```python
from build123d import *

# Parameters (mm, degrees)
EXTRUDE_1_DEPTH     = 35
FILLET_START        = -36
FILLET_1_DEPTH      = 37
FILLET_START_2      = -35
FILLET_1_2_DEPTH    = 35
SKETCH_2_R          = 2
CUT_EXTRUDE_1_DEPTH = 40.515819617
CUT_EXTRUDE_2_DEPTH = 2.5
EXTRUDE_2_DEPTH     = 5.1


with BuildPart() as part:
    # 草图1 → 凸台-拉伸1 (new body)
    with BuildSketch(Plane.XY):
        with BuildLine():
            Line((-2, 11.5), (-2, -11.5))
            Line((-2, -11.5), (0, -11.5))
            Line((0, -11.5), (0, -14.5))
            Line((0, -14.5), (0, -17.5))
            Line((0, -17.5), (-1, -17.5))
            Line((-1, -17.5), (-1, -14.5))
            ThreePointArc((-1, -14.5), (-1.292893219, -13.792893219), (-2, -13.5))
            Line((-2, -13.5), (-3.5, -13.5))
            ThreePointArc((-3.5, -13.5), (-4.914213562, -12.914213562), (-5.5, -11.5))
            Line((-5.5, -11.5), (-5.5, 11.5))
            ThreePointArc((-5.5, 11.5), (-4.914213562, 12.914213562), (-3.5, 13.5))
            Line((-3.5, 13.5), (-2, 13.5))
            ThreePointArc((-2, 13.5), (-1.292893219, 13.792893219), (-1, 14.5))
            Line((-1, 14.5), (-1, 17.5))
            Line((-1, 17.5), (0, 17.5))
            Line((0, 17.5), (0, 14.5))
            Line((0, 14.5), (0, 11.5))
            Line((0, 11.5), (-2, 11.5))
        make_face()
    extrude(amount=-EXTRUDE_1_DEPTH)

    # 圆角1: read off the stored shape, not the designer's step
    # 圆角1 outline → 圆角1 (cut)
    with BuildSketch(Plane.XY.offset(FILLET_START)):
        with BuildLine():
            Line((0, -11.5), (-1, -11.5))
            ThreePointArc((-1, -11.5), (-0.292893219, -11.792893219), (0, -12.5))
            Line((0, -12.5), (0, -11.5))
        make_face()
        with BuildLine():
            ThreePointArc((0, 12.5), (-0.292893219, 11.792893219), (-1, 11.5))
            Line((-1, 11.5), (0, 11.5))
            Line((0, 11.5), (0, 12.5))
        make_face()
    extrude(amount=FILLET_1_DEPTH, mode=Mode.SUBTRACT)

    # Fillet 1 2 outline → Fillet 1 2 (add)
    with BuildSketch(Plane.XY.offset(FILLET_START_2)):
        with BuildLine():
            Line((-2, -11.5), (-1, -11.5))
            ThreePointArc((-1, -11.5), (-1.707106781, -11.207106781), (-2, -10.5))
            Line((-2, -10.5), (-2, -11.5))
        make_face()
        with BuildLine():
            Line((-2, 11.5), (-2, 10.5))
            ThreePointArc((-2, 10.5), (-1.707106781, 11.207106781), (-1, 11.5))
            Line((-1, 11.5), (-2, 11.5))
        make_face()
    extrude(amount=FILLET_1_2_DEPTH)

    # 草图2 → 切除-拉伸1 (cut, through all)
    with BuildSketch(Plane.ZY.offset(5.5)):
        with Locations(Location((-17.5, 0, 0), (0, 0, 270))):
            Circle(SKETCH_2_R)
    extrude(amount=-CUT_EXTRUDE_1_DEPTH, mode=Mode.SUBTRACT)

    # 草图3 → 切除-拉伸2 (cut)
    with BuildSketch(Plane(origin=(-2, 0, 0), x_dir=(0, 0, -1), z_dir=(1, 0, 0))):
        Polygon((19.15, -2.857883832), (20.8, 0), (19.15, 2.857883832), (15.85, 2.857883832), (14.2, 0), (15.85, -2.857883832), align=None)
    extrude(amount=-CUT_EXTRUDE_2_DEPTH, mode=Mode.SUBTRACT)

    # 草图4 → 凸台-拉伸2 (add)
    with BuildSketch(Plane.ZY.offset(5.5)):
        with BuildLine():
            Line((-3.055300855, -4.891227974), (-3.100019781, 4.908669996))
            ThreePointArc((-3.100019781, 4.908669996), (-5, 6.8), (-6.899980219, 4.908669996))
            Line((-6.899980219, 4.908669996), (-6.944699145, -4.891227974))
            ThreePointArc((-6.944699145, -4.891227974), (-5, -6.844821423), (-3.055300855, -4.891227974))
        make_face()
        with BuildLine():
            Line((-31.899980219, 4.908669996), (-31.944699145, -4.891227974))
            ThreePointArc((-31.944699145, -4.891227974), (-30, -6.844821423), (-28.055300855, -4.891227974))
            Line((-28.055300855, -4.891227974), (-28.100019781, 4.908669996))
            ThreePointArc((-28.100019781, 4.908669996), (-30, 6.8), (-31.899980219, 4.908669996))
        make_face()
    extrude(amount=EXTRUDE_2_DEPTH)


solid = part.part
```
Model file for the job. Use its own axes, mm. A direction names the side the tool comes from. Coordinates: 2 decimals unless noted, no trailing zeros. Order: outer loops, then holes, each group sorted by start corner. A loop starts at its lowest first (then second) coordinate and runs counter-clockwise, first axis right, second up. Notation, with made-up numbers: (36, 71.5) -> (72, 71.5) arc R28 ccw to (72, 96.5) -> close; hole circle Ø11 at (-13.5, 64.5). An arc over 180 degrees is marked (long way). Return JSON: item names as keys, results as strings.
Item 1: Mould opens along Y. For faces 6 (the face through (-2, 0, -21)), 7 (the face through (-3.232, 1.409, -19.987)), 8 (the face through (-0.5, -17.5, -17.3)), 9 (the face through (-5.5, -3, -17)) say: pulls with the +Y half, pulls with the -Y half, needs draft (parallel to the pull), parting line crosses it, or undercut.
Model answer:
{"face 6": "undercut", "face 7": "undercut", "face 8": "pulls with the -Y half", "face 9": "needs draft"}
Item 2: Slice it at C-C (x = -2.5). Write the cut outline in (y, z).
Model answer:
{"outline": "(-13.5, -35) -> (13.5, -35) -> (13.5, 0) -> (-13.5, 0) -> close; hole (-2.86, -19.15) -> (0, -20.8) -> (2.86, -19.15) -> (2.86, -15.85) -> (0, -14.2) -> (-2.86, -15.85) -> close"}
Item 3: Slice it at A-A (x = -6). Write the cut outline in (y, z).
Model answer:
{"outline": "(-4.89, -31.94) -> (4.91, -31.9) arc R1.9 ccw to (4.91, -28.1) -> (-4.89, -28.06) arc R1.94 ccw (long way) to start; (-4.89, -6.94) -> (4.91, -6.9) arc R1.9 ccw to (4.91, -3.1) -> (-4.89, -3.06) arc R1.94 ccw (long way) to start"}
Item 4: Slice it at D-D (z = -30). Write the cut outline in (x, y).
Model answer:
{"outline": "(-10.6, -6.84) -> (-5.5, -6.84) -> (-5.5, -11.5) arc R2 ccw to (-3.5, -13.5) -> (-2, -13.5) arc R1 cw to (-1, -14.5) -> (-1, -17.5) -> (0, -17.5) -> (0, -12.5) arc R1 ccw to (-1, -11.5) arc R1 cw to (-2, -10.5) -> (-2, 10.5) arc R1 cw to (-1, 11.5) arc R1 ccw to (0, 12.5) -> (0, 17.5) -> (-1, 17.5) -> (-1, 14.5) arc R1 cw to (-2, 13.5) -> (-3.5, 13.5) arc R2 ccw to (-5.5, 11.5) -> (-5.5, 6.8) -> (-10.6, 6.8) -> close"}
Item 5: 3-axis set-ups, long thin cutter, end or side, ignore diameter. For faces 1 (the face through (-3, 13.5, -17)), 2 (the face through (-8, 6.8, -30)), 3 (the face through (-3.232, -1.409, -15.013)), 4 (the face through (-10.6, 0, -5)), 5 (the face through (-3, -13.5, -17)): which of +Z, -Z, +X, -X, +Y, -Y reach the whole face in a straight line?
Model answer:
{"face 1": "+Z, -Z, -X, +Y", "face 2": "-X, +Y", "face 3": "+X", "face 4": "+Z, -Z, -X, +Y, -Y", "face 5": "+Z, -Z, -X, -Y"}
Item 6: Wall check: line 1 along Z through (x, y) = (-6, 4.5); line 2 along Z through (x, y) = (-5.1, 0); line 3 along X through (y, z) = (15, -26.5). Give the ranges that are in metal, low to high. Write a range as from..to.
Model answer:
{"line 1": "z = -31.9..-28.1, -6.9..-3.1", "line 2": "z = -35..-19.5, -15.5..0", "line 3": "x = -1..0"}
Item 7: Slice it at B-B (z = -17.5). Write the cut outline in (x, y), then the cut area to 3 significant figures.
Model answer:
{"outline": "(-5.5, -11.5) arc R2 ccw to (-3.5, -13.5) -> (-2, -13.5) arc R1 cw to (-1, -14.5) -> (-1, -17.5) -> (0, -17.5) -> (0, -12.5) arc R1 ccw to (-1, -11.5) arc R1 cw to (-2, -10.5) -> (-2, -2.86) -> (-4.5, -2.86) -> (-4.5, -2) -> (-5.5, -2) -> close; (-5.5, 2) -> (-4.5, 2) -> (-4.5, 2.86) -> (-2, 2.86) -> (-2, 10.5) arc R1 cw to (-1, 11.5) arc R1 ccw to (0, 12.5) -> (0, 17.5) -> (-1, 17.5) -> (-1, 14.5) arc R1 cw to (-2, 13.5) -> (-3.5, 13.5) arc R2 ccw to (-5.5, 11.5) -> close", "area": "90.9 mm²"}
Item 8: Pin check, flat tips, straight feed: P1, Ø1.2, axis at x = -2.5, z = -20.5, coming from the -Y side (3 decimals); P2, Ø1.6, axis at x = -2.5, z = -13, coming from the +Y side; P3, Ø6.5, axis at y = 0, z = -17.5, coming from the -X side. Stop position of each tip, or through.
Model answer:
{"P1": "stops at y = -13.505", "P2": "stops at y = 13.55", "P3": "stops at x = -5.5"}
